```python
from build123d import *

# Parameters (mm, degrees)
SKETCH1_R           = 15.875
SKETCH1_R_2         = 12.7
BOSS_EXTRUDE1_DEPTH = 100
SKETCH2_R           = 2.1
CUT_EXTRUDE1_DEPTH  = 103.489176258
CIRPATTERN1_COUNT   = 6


with BuildPart() as part:
    # Sketch1 → Boss-Extrude1 (new, symmetric)
    with BuildSketch(Plane(origin=(0, 0, 0), x_dir=(1, 0, 0), z_dir=(0, 1, 0))):
        with Locations(Location((0, 0, 0), (0, 0, 270))):
            Circle(SKETCH1_R)
        with Locations(Location((0, 0, 0), (0, 0, 270))):
            Circle(SKETCH1_R_2, mode=Mode.SUBTRACT)
    extrude(amount=BOSS_EXTRUDE1_DEPTH, both=True)

    # Sketch2 → Cut-Extrude1 (cut, through all)
    with BuildSketch(Plane.XY):
        with Locations(Location((0, -95.5, 0), (0, 0, 90))):
            Circle(SKETCH2_R)
    cut_extrude1 = extrude(amount=-CUT_EXTRUDE1_DEPTH, mode=Mode.SUBTRACT)

    # CirPattern1: Cut-Extrude1 ×6 about axis
    cirpattern1_axis = Axis((0, 100, 0), (0, -1, 0))
    for i in range(1, CIRPATTERN1_COUNT):
        add(cut_extrude1.rotate(cirpattern1_axis, i * 360 / CIRPATTERN1_COUNT), mode=Mode.SUBTRACT)


solid = part.part
```
Verification items for the finished model (mm, model axes). Give positions to 0.01 mm unless a question says otherwise; leave off trailing zeros. Order: outer loops, then holes, each group sorted by start corner. A loop starts at its lowest first (then second) coordinate and runs counter-clockwise, first axis right, second up. Notation, with made-up numbers: (51.25, 58.25) -> (92.25, 58.25) arc R16 ccw to (92.25, 73.25) -> close; hole circle Ø8 at (50.25, 34.5). An arc over 180 degrees is marked (long way). Use a Markdown table: item, result.
1) Mould release check, pull along Y, two halves, no side actions. Record for faces 1 (the flat face through (11, 100, -7)), 2 (the cylindrical face through (-12.68, -93.56, 6.39)), 3 (the cylindrical face through (-0.8, -93.56, 14.18)), 4 (the flat face through (11, -100, -7)): pulls with the +Y half, pulls with the -Y half, needs draft (parallel to the pull), parting line crosses it, or undercut.
Results:
| item | result |
|---|---|
| face 1 | pulls with the +Y half |
| face 2 | undercut |
| face 3 | undercut |
| face 4 | pulls with the -Y half |
2) Material ranges on probe 1 along X at (y, z) = (-37, 0) (3 decimals); probe 2 along Y at (x, z) = (0, 14.25); probe 3 along Z at (x, y) = (1, 47.5), recorded low to high.
Results:
| item | result |
|---|---|
| probe 1 | -15.875 to -12.7, 12.7 to 15.875 |
| probe 2 | -100 to -97.6, -93.4 to 100 |
| probe 3 | -15.84 to -12.66, 12.66 to 15.84 |
3) Section check B-B, the plane z = 0. Record the boundary of the cut face in (x, y) (3 decimals).
Results:
| item | result |
|---|---|
| outline | (-15.875, -100) -> (-12.7, -100) -> (-12.7, 100) -> (-15.875, 100) -> close; (12.7, -100) -> (15.875, -100) -> (15.875, 100) -> (12.7, 100) -> close |
4) Depth check by flat-ended pin: pin 1 Ø2.5 at (x, y) = (0, -95.5) entering from +Z; pin 2 Ø3 at (y, z) = (-72.5, -2) entering from +X; pin 3 Ø3 at (y, z) = (-57.5, -7) entering from -X; pin 4 Ø12 at (y, z) = (61.5, -7.5) entering from -X. Enter the tip coordinate at first touch or a pass-through.
Results:
| item | result |
|---|---|
| pin 1 | through |
| pin 2 | x = 15.87 |
| pin 3 | x = -14.89 |
| pin 4 | x = -15.8 |
5) Section check D-D, the plane y = 28. Record the boundary of the cut face in (x, z) (3 decimals).
Results:
| item | result |
|---|---|
| outline | circle Ø31.75 at (0, 0); hole circle Ø25.4 at (0, 0) |
6) Section check A-A, the plane x = 0. Record the boundary of the cut face in (y, z) (3 decimals), then the cut area to 3 significant figures.
Results:
| item | result |
|---|---|
| outline | (-100, -15.875) -> (-97.6, -15.875) -> (-97.6, -12.7) -> (-100, -12.7) -> close; (-100, 12.7) -> (-97.6, 12.7) -> (-97.6, 15.875) -> (-100, 15.875) -> close; (-93.4, -15.875) -> (100, -15.875) -> (100, -12.7) -> (-93.4, -12.7) -> close; (-93.4, 12.7) -> (100, 12.7) -> (100, 15.875) -> (-93.4, 15.875) -> close |
| area | 1,240 mm² |
7) Section check C-C, the plane y = -95.5. Record the boundary of the cut face in (x, z) (3 decimals), then the cut area to 3 significant figures.
Results:
| item | result |
|---|---|
| outline | (-14.677, -6.049) -> (-11.897, -4.444) arc R12.7 cw to (-11.897, 4.444) -> (-14.677, 6.049) arc R15.875 ccw to start; (-12.577, -9.686) arc R15.875 ccw to (-2.1, -15.735) -> (-2.1, -12.525) arc R12.7 cw to (-9.797, -8.081) -> close; (-12.577, 9.686) -> (-9.797, 8.081) arc R12.7 cw to (-2.1, 12.525) -> (-2.1, 15.735) arc R15.875 ccw to start; (2.1, -15.735) arc R15.875 ccw to (12.577, -9.686) -> (9.797, -8.081) arc R12.7 cw to (2.1, -12.525) -> close; (2.1, 12.525) arc R12.7 cw to (9.797, 8.081) -> (12.577, 9.686) arc R15.875 ccw to (2.1, 15.735) -> close; (11.897, -4.444) -> (14.677, -6.049) arc R15.875 ccw to (14.677, 6.049) -> (11.897, 4.444) arc R12.7 cw to start |
| area | 205 mm² |
